```python
from build123d import *

# Parameters (mm, degrees)
SZKIC1_W                    = 95.25
SZKIC1_H                    = 60
DODANIE_WYCI_GNI_CIE1_DEPTH = 10
SZKIC2_W                    = 93
SZKIC2_H                    = 57.5
WYTNIJ_WYCI_GNI_CIE1_DEPTH  = 9
DODANIE_WYCI_GNI_CIE3_DEPTH = 60
WYTNIJ_WYCI_GNI_CIE2_REACH  = 106.318
DODANIE_WYCI_GNI_CIE4_DEPTH = 1
ZAOKR_GLENIE1_R             = 0.63
ZAOKR_GLENIE2_R             = 5
ZAOKR_GLENIE3_R             = 0.5
DODANIE_WYCI_GNI_CIE2_DEPTH = 4.5
ZAOKR_GLENIE4_R             = 4


with BuildPart() as part:
    # Szkic1 → Dodanie-wyciągnięcie1 (new body)
    with BuildSketch(Plane.XY):
        with Locations((0.125, 0)):
            Rectangle(SZKIC1_W, SZKIC1_H)
    extrude(amount=DODANIE_WYCI_GNI_CIE1_DEPTH)

    # Szkic2 → Wytnij-wyciągnięcie1 (cut)
    with BuildSketch(Plane.XY.offset(10)):
        Rectangle(SZKIC2_W, SZKIC2_H)
    extrude(amount=-WYTNIJ_WYCI_GNI_CIE1_DEPTH, mode=Mode.SUBTRACT)

    # Szkic4 → Dodanie-wyciągnięcie3 (add)
    with BuildSketch(Plane.XY):
        with BuildLine():
            Line((-46.5, -30), (-74.192307692, -18.461538462))
            ThreePointArc((-74.192307692, -18.461538462), (-86.5, 0), (-74.192307692, 18.461538462))
            Line((-74.192307692, 18.461538462), (-46.5, 30))
            Line((-46.5, 30), (-46.5, -30))
        make_face()
        with BuildLine():
            Line((-47.5, -28.5), (-73.807692308, -17.538461538))
            ThreePointArc((-73.807692308, -17.538461538), (-85.5, 0), (-73.807692308, 17.538461538))
            Line((-73.807692308, 17.538461538), (-47.5, 28.5))
            Line((-47.5, 28.5), (-47.5, -28.5))
        make_face(mode=Mode.SUBTRACT)
    extrude(amount=DODANIE_WYCI_GNI_CIE3_DEPTH)

    # Szkic6 → Wytnij-wyciągnięcie2 (cut, up to next)
    with BuildSketch(Plane.XY.offset(10), mode=Mode.PRIVATE) as wytnij_wyci_gni_cie2_sk1:
        Polygon((-46.5, -30), (-47.5, -29.583333333), (-47.5, -30), align=None)
    wytnij_wyci_gni_cie2_tool1 = extrude(wytnij_wyci_gni_cie2_sk1.sketch, amount=-WYTNIJ_WYCI_GNI_CIE2_REACH, mode=Mode.PRIVATE) & part.part
    # Szkic6 → Wytnij-wyciągnięcie2 (cut, up to next)
    with BuildSketch(Plane.XY.offset(10), mode=Mode.PRIVATE) as wytnij_wyci_gni_cie2_sk2:
        Polygon((-46.5, 30), (-47.5, 29.583333333), (-47.5, 30), align=None)
    wytnij_wyci_gni_cie2_tool2 = extrude(wytnij_wyci_gni_cie2_sk2.sketch, amount=-WYTNIJ_WYCI_GNI_CIE2_REACH, mode=Mode.PRIVATE) & part.part
    add(wytnij_wyci_gni_cie2_tool1.solids().sort_by_distance((-47.166667, -29.861111, 10))[0], mode=Mode.SUBTRACT)
    add(wytnij_wyci_gni_cie2_tool2.solids().sort_by_distance((-47.166667, 29.861111, 10))[0], mode=Mode.SUBTRACT)

    # Szkic5 → Dodanie-wyciągnięcie4 (add)
    with BuildSketch(Plane(origin=(0, 0, 0), x_dir=(-1, 0, 0), z_dir=(0, 0, -1))):
        with BuildLine():
            Line((73.807692308, -17.538461538), (47.5, -28.5))
            Line((47.5, -28.5), (47.5, 28.5))
            Line((47.5, 28.5), (73.807692308, 17.538461538))
            ThreePointArc((73.807692308, 17.538461538), (85.5, 0), (73.807692308, -17.538461538))
        make_face()
    extrude(amount=-DODANIE_WYCI_GNI_CIE4_DEPTH)

    # Zaokrąglenie1
    # the kernel refuses this fillet: 0.63 mm, written as the material it takes off along each edge
    with BuildSketch(Plane(origin=(47.12, 29.37, 9.37), x_dir=(1, 0, 0), z_dir=(0, 1, 0))) as zaokr_glenie1_piece_1_section:
        Polygon((0, 0), (ZAOKR_GLENIE1_R * 1.02, 0), (ZAOKR_GLENIE1_R * 1.02, -ZAOKR_GLENIE1_R * 1.02), (0, -ZAOKR_GLENIE1_R * 1.02), align=None)
    zaokr_glenie1_piece_1 = extrude(amount=ZAOKR_GLENIE1_R * 1.02, mode=Mode.PRIVATE)
    zaokr_glenie1_piece_1 = zaokr_glenie1_piece_1 - Plane(origin=(47.12, 29.37, 9.37), x_dir=(-0.7071067811865475, 0, -0.7071067811865475), z_dir=(0, 1, 0)) * Sphere(ZAOKR_GLENIE1_R, mode=Mode.PRIVATE)
    add(zaokr_glenie1_piece_1, mode=Mode.SUBTRACT)
    with BuildSketch(Plane(origin=(47.12, -29.37, 9.37), x_dir=(0, 0, 1), z_dir=(1, 0, 0))) as zaokr_glenie1_piece_2_section:
        Polygon((0, 0), (ZAOKR_GLENIE1_R * 1.02, 0), (ZAOKR_GLENIE1_R * 1.02, ZAOKR_GLENIE1_R * 1.02), (0, ZAOKR_GLENIE1_R * 1.02), align=None)
    zaokr_glenie1_piece_2 = extrude(amount=ZAOKR_GLENIE1_R * 1.02, mode=Mode.PRIVATE)
    zaokr_glenie1_piece_2 = zaokr_glenie1_piece_2 - Plane(origin=(47.12, -29.37, 9.37), x_dir=(0, 0.7071067811865475, -0.7071067811865475), z_dir=(1, 0, 0)) * Sphere(ZAOKR_GLENIE1_R, mode=Mode.PRIVATE)
    add(zaokr_glenie1_piece_2, mode=Mode.SUBTRACT)
    with BuildSketch(Plane(origin=(47.75, 30, -1.575), x_dir=(-1, 0, 0), z_dir=(0, 0, 1)), Plane(origin=(47.75, -30, -1.575), x_dir=(0, 1, 0), z_dir=(0, 0, 1))) as zaokr_glenie1_piece_3:
        with BuildLine():
            CenterArc((ZAOKR_GLENIE1_R, ZAOKR_GLENIE1_R), ZAOKR_GLENIE1_R, 180, 90)
            Line((0, ZAOKR_GLENIE1_R), (0, 0))
            Line((0, 0), (ZAOKR_GLENIE1_R, 0))
        make_face()
    extrude(amount=10.945, mode=Mode.SUBTRACT)
    with BuildSketch(Plane(origin=(-46.5, 30, 10), x_dir=(0, 0, -1), z_dir=(1, 0, 0))) as zaokr_glenie1_piece_4:
        with BuildLine():
            CenterArc((ZAOKR_GLENIE1_R, -ZAOKR_GLENIE1_R), ZAOKR_GLENIE1_R, 90, 90)
            Line((0, -ZAOKR_GLENIE1_R), (0, 0))
            Line((0, 0), (ZAOKR_GLENIE1_R, 0))
        make_face()
    extrude(amount=93.62, mode=Mode.SUBTRACT)
    with BuildSketch(Plane(origin=(47.75, 29.37, 10), x_dir=(0, 0, -1), z_dir=(0, -1, 0))) as zaokr_glenie1_piece_5:
        with BuildLine():
            CenterArc((ZAOKR_GLENIE1_R, -ZAOKR_GLENIE1_R), ZAOKR_GLENIE1_R, 90, 90)
            Line((0, -ZAOKR_GLENIE1_R), (0, 0))
            Line((0, 0), (ZAOKR_GLENIE1_R, 0))
        make_face()
    extrude(amount=58.74, mode=Mode.SUBTRACT)
    with BuildSketch(Plane(origin=(47.12, -30, 10), x_dir=(0, 1, 0), z_dir=(-1, 0, 0))) as zaokr_glenie1_piece_6:
        with BuildLine():
            CenterArc((ZAOKR_GLENIE1_R, ZAOKR_GLENIE1_R), ZAOKR_GLENIE1_R, 180, 90)
            Line((0, ZAOKR_GLENIE1_R), (0, 0))
            Line((0, 0), (ZAOKR_GLENIE1_R, 0))
        make_face()
    extrude(amount=93.62, mode=Mode.SUBTRACT)
    with BuildSketch(Plane(origin=(46.5, 28.75, 10), x_dir=(1, 0, 0), z_dir=(0, -1, 0))) as zaokr_glenie1_piece_7:
        with BuildLine():
            CenterArc((ZAOKR_GLENIE1_R, -ZAOKR_GLENIE1_R), ZAOKR_GLENIE1_R, 90, 90)
            Line((0, -ZAOKR_GLENIE1_R), (0, 0))
            Line((0, 0), (ZAOKR_GLENIE1_R, 0))
        make_face()
    extrude(amount=57.5, mode=Mode.SUBTRACT)
    with BuildSketch(Plane(origin=(-46.5, 28.75, 10), x_dir=(0, 1, 0), z_dir=(1, 0, 0)), Plane(origin=(46.5, -28.75, 10), x_dir=(0, -1, 0), z_dir=(-1, 0, 0))) as zaokr_glenie1_piece_8:
        with BuildLine():
            CenterArc((ZAOKR_GLENIE1_R, -ZAOKR_GLENIE1_R), ZAOKR_GLENIE1_R, 90, 90)
            Line((0, -ZAOKR_GLENIE1_R), (0, 0))
            Line((0, 0), (ZAOKR_GLENIE1_R, 0))
        make_face()
    extrude(amount=93, mode=Mode.SUBTRACT)
    with BuildSketch(Plane(origin=(-46.5, 28.75, 10), x_dir=(0, 1, 0), z_dir=(1, 0, 0))) as zaokr_glenie1_piece_9a_section:
        with BuildLine():
            CenterArc((ZAOKR_GLENIE1_R, -ZAOKR_GLENIE1_R), ZAOKR_GLENIE1_R, 90, 90)
            Line((0, -ZAOKR_GLENIE1_R), (0, 0))
            Line((0, 0), (ZAOKR_GLENIE1_R, 0))
        make_face()
    zaokr_glenie1_piece_9a = extrude(amount=94.575, mode=Mode.PRIVATE)
    zaokr_glenie1_piece_9a = split(zaokr_glenie1_piece_9a, bisect_by=Plane(origin=(47.75, 28.75, 10), z_dir=(-1, 0, 0)), keep=Keep.TOP, mode=Mode.PRIVATE)
    zaokr_glenie1_piece_9a = split(zaokr_glenie1_piece_9a, bisect_by=Plane(origin=(46.5, 28.75, 10), z_dir=(1, 0, 0)), keep=Keep.TOP, mode=Mode.PRIVATE)
    with BuildSketch(Plane(origin=(46.5, 30.325, 10), x_dir=(1, 0, 0), z_dir=(0, -1, 0))) as zaokr_glenie1_piece_9b_section:
        with BuildLine():
            CenterArc((ZAOKR_GLENIE1_R, -ZAOKR_GLENIE1_R), ZAOKR_GLENIE1_R, 90, 90)
            Line((0, -ZAOKR_GLENIE1_R), (0, 0))
            Line((0, 0), (ZAOKR_GLENIE1_R, 0))
        make_face()
    zaokr_glenie1_piece_9b = extrude(amount=59.075, mode=Mode.PRIVATE)
    zaokr_glenie1_piece_9b = split(zaokr_glenie1_piece_9b, bisect_by=Plane(origin=(46.5, 30, 10), z_dir=(0, -1, 0)), keep=Keep.TOP, mode=Mode.PRIVATE)
    zaokr_glenie1_piece_9b = split(zaokr_glenie1_piece_9b, bisect_by=Plane(origin=(46.5, 28.75, 10), z_dir=(0, 1, 0)), keep=Keep.TOP, mode=Mode.PRIVATE)
    zaokr_glenie1_piece_9 = zaokr_glenie1_piece_9a & zaokr_glenie1_piece_9b
    add(zaokr_glenie1_piece_9, mode=Mode.SUBTRACT)
    with BuildSketch(Plane(origin=(46.5, 28.75, 10), x_dir=(1, 0, 0), z_dir=(0, -1, 0))) as zaokr_glenie1_piece_10a_section:
        with BuildLine():
            CenterArc((ZAOKR_GLENIE1_R, -ZAOKR_GLENIE1_R), ZAOKR_GLENIE1_R, 90, 90)
            Line((0, -ZAOKR_GLENIE1_R), (0, 0))
            Line((0, 0), (ZAOKR_GLENIE1_R, 0))
        make_face()
    zaokr_glenie1_piece_10a = extrude(amount=59.075, mode=Mode.PRIVATE)
    zaokr_glenie1_piece_10a = split(zaokr_glenie1_piece_10a, bisect_by=Plane(origin=(46.5, -30, 10), z_dir=(0, 1, 0)), keep=Keep.TOP, mode=Mode.PRIVATE)
    zaokr_glenie1_piece_10a = split(zaokr_glenie1_piece_10a, bisect_by=Plane(origin=(46.5, -28.75, 10), z_dir=(0, -1, 0)), keep=Keep.TOP, mode=Mode.PRIVATE)
    with BuildSketch(Plane(origin=(48.075, -28.75, 10), x_dir=(0, -1, 0), z_dir=(-1, 0, 0))) as zaokr_glenie1_piece_10b_section:
        with BuildLine():
            CenterArc((ZAOKR_GLENIE1_R, -ZAOKR_GLENIE1_R), ZAOKR_GLENIE1_R, 90, 90)
            Line((0, -ZAOKR_GLENIE1_R), (0, 0))
            Line((0, 0), (ZAOKR_GLENIE1_R, 0))
        make_face()
    zaokr_glenie1_piece_10b = extrude(amount=94.575, mode=Mode.PRIVATE)
    zaokr_glenie1_piece_10b = split(zaokr_glenie1_piece_10b, bisect_by=Plane(origin=(47.75, -28.75, 10), z_dir=(-1, 0, 0)), keep=Keep.TOP, mode=Mode.PRIVATE)
    zaokr_glenie1_piece_10b = split(zaokr_glenie1_piece_10b, bisect_by=Plane(origin=(46.5, -28.75, 10), z_dir=(1, 0, 0)), keep=Keep.TOP, mode=Mode.PRIVATE)
    zaokr_glenie1_piece_10 = zaokr_glenie1_piece_10a & zaokr_glenie1_piece_10b
    add(zaokr_glenie1_piece_10, mode=Mode.SUBTRACT)

    # Zaokrąglenie2
    zaokr_glenie2_edges = [part.edges().sort_by_distance(p)[0] for p in [
        (-47.5, 28.5, 30.5),
        (-47.5, -28.5, 30.5),
    ]]
    fillet(zaokr_glenie2_edges, radius=ZAOKR_GLENIE2_R)

    # Zaokrąglenie3
    zaokr_glenie3_edges = [part.edges().sort_by_distance(p)[0] for p in [
        (-86.5, 0, 60),
        (-60.346153846, -24.230769231, 60),
        (-46.5, 0, 60),
        (-60.346153846, 24.230769231, 60),
    ]]
    fillet(zaokr_glenie3_edges, radius=ZAOKR_GLENIE3_R)

    # Szkic3 → Dodanie-wyciągnięcie2 (add)
    with BuildSketch(Plane.XY.offset(1)):
        Polygon((46.5, -28.75), (46.5, -24.75), (42.5, -28.75), align=None)
        Polygon((-42.5, -28.75), (-46.5, -28.75), (-46.5, -24.75), align=None)
        Polygon((-46.5, 28.75), (-46.5, 24.75), (-42.5, 28.75), align=None)
        Polygon((42.5, 28.75), (46.5, 28.75), (46.5, 24.75), align=None)
    extrude(amount=DODANIE_WYCI_GNI_CIE2_DEPTH)

    # Zaokrąglenie4
    zaokr_glenie4_edges = [part.edges().sort_by_distance(p)[0] for p in [
        (-47.5, 0, 1),
        (-64.115384615, -21.576923077, 1),
        (-49.726499019, -25.160251472, 1),
        (-49.726499019, 25.160251472, 1),
        (-85.5, 0, 1),
        (-64.115384615, 21.576923077, 1),
    ]]
    fillet(zaokr_glenie4_edges, radius=ZAOKR_GLENIE4_R)


solid = part.part
```
Check sheet for the modelled part. Datum: model origin and axes. Units: mm. A direction names the side the tool comes from. Coordinates: 2 decimals unless noted, no trailing zeros. Loops run counter-clockwise (first coordinate to the right, second up) from the corner with the lowest first, then second, coordinate; pieces in that order, holes last. Notation, with made-up numbers: M 78.5,26.25 L 133.5,26.25 A24 ccw 133.5,64.25 Z; hole C 65.25,2 d7. An arc over 180 degrees is marked long. Answer as a JSON object with one key per item and string values.
1. Release check for a two-part mould opening along Y. For faces 3 (the flat face through (47.75, 0, 5)), 4 (the flat face through (0, -30, 5)), 5 (the flat face through (-44.53, 26.72, 3.22)) record: pulls with the +Y half, pulls with the -Y half, needs draft (parallel to the pull), parting line crosses it, or undercut.
Outcome:
{"face 3": "needs draft", "face 4": "pulls with the -Y half", "face 5": "undercut"}
2. Sectioned sample at B-B on z = 7. Record the cut outline in (x, y), and give its area (3 significant figures).
Outcome:
{"outline": "M -74.19,-18.46 L -46.5,-30 L 47.12,-30 A0.63 ccw 47.75,-29.37 L 47.75,29.37 A0.63 ccw 47.12,30 L -46.5,30 L -74.19,18.46 A20 ccw Z; hole M -73.81,-17.54 L -54.42,-25.62 A5 ccw -47.5,-21 L -47.5,21 A5 ccw -54.42,25.62 L -73.81,17.54 A19 ccw Z; hole M -46.5,-28.75 L 46.5,-28.75 L 46.5,28.75 L -46.5,28.75 Z", "area": "496 mm²"}
3. Access from +Z, -Z, +X, -X, +Y, -Y to the whole of each face (thin tool, end or side, straight path). Record for faces 1 (the flat face through (-1, -28.75, 5)), 2 (the flat face through (0, 30, 5)).
Outcome:
{"face 1": "+Z", "face 2": "+Z, -Z, +X, -X, +Y"}
4. Depth check by flat-ended pin: P1, Ø2, axis at x = -43.5, y = -26, coming from the +Z side; P2, Ø2, axis at x = 44.5, y = -26, coming from the +Z side; P3, Ø2, axis at y = -9.5, z = 21.5, coming from the +X side. Enter the tip coordinate at first touch or a pass-through.
Outcome:
{"P1": "z = 1", "P2": "z = 5.5", "P3": "x = -46.5"}
5. Sectioned sample at A-A on z = 34. Record the cut outline in (x, y).
Outcome:
{"outline": "M -74.19,-18.46 L -46.5,-30 L -46.5,30 L -74.19,18.46 A20 ccw Z; hole M -73.81,-17.54 L -54.42,-25.62 A5 ccw -47.5,-21 L -47.5,21 A5 ccw -54.42,25.62 L -73.81,17.54 A19 ccw Z"}
6. Sectioned sample at C-C on x = -23.5. Record the cut outline in (y, z) (3 decimals), and give its area (3 significant figures).
Outcome:
{"outline": "M -30,0 L 30,0 L 30,9.37 A0.63 ccw 29.375,10 A0.63 ccw 28.75,9.37 L 28.75,1 L -28.75,1 L -28.75,9.37 A0.63 ccw -29.375,10 A0.63 ccw -30,9.37 Z", "area": "82.2 mm²"}
7. Scan lines: L1, parallel to X at y = -1, z = 6; L2, parallel to X at y = -12, z = 9.5; L3, parallel to Z at x = -72.5, y = -2.5. Record each from-to range of solid material in increasing order. Write a range as from..to.
Outcome:
{"L1": "-86.47..-85.47, -47.5..-46.5, 46.5..47.75", "L2": "-82.5..-81.23, -47.5..-46.5, 46.51..47.74", "L3": "0..1"}
